```python
from build123d import *

# Parameters (mm, degrees)
SKETCH1_R           = 1.65
BOSS_EXTRUDE1_DEPTH = 2
SKETCH2_R           = 1.25
BOSS_EXTRUDE2_DEPTH = 2
SKETCH3_R           = 7.5
CUT_EXTRUDE1_DEPTH  = 2
BOSS_EXTRUDE3_START = 2.65408
SKETCH4_R           = 2.5
SKETCH4_R_2         = 1.25
BOSS_EXTRUDE3_DEPTH = 2.65408
SKETCH5_R           = 1.797788616
SKETCH5_R_2         = 1.10000034
SKETCH5_R_3         = 2.012466026
SKETCH5_R_4         = 1.729091626
SKETCH5_R_5         = 1.81324602
SKETCH5_R_6         = 1.075
BOSS_EXTRUDE4_DEPTH = 4.65408
CHAMFER1_SIZE       = 1.714507845
CHAMFER1_SIZE_2     = 0.15


with BuildPart() as part:
    # Sketch1 → Boss-Extrude1 (new body)
    with BuildSketch(Plane.XY):
        with BuildLine():
            Line((24.04163056, 18.384776311), (9.309167823, 3.652313574))
            ThreePointArc((9.309167823, 3.652313574), (9.985739131, -0.533867035), (8.866689125, -4.624048438))
            Line((8.866689125, -4.624048438), (23.334523779, -19.091883092))
            ThreePointArc((23.334523779, -19.091883092), (23.334523779, -23.334523779), (19.091883092, -23.334523779))
            Line((19.091883092, -23.334523779), (4.624048438, -8.866689125))
            ThreePointArc((4.624048438, -8.866689125), (0.533867035, -9.985739131), (-3.652313574, -9.309167823))
            Line((-3.652313574, -9.309167823), (-18.384776311, -24.04163056))
            ThreePointArc((-18.384776311, -24.04163056), (-24.04163056, -24.04163056), (-24.04163056, -18.384776311))
            Line((-24.04163056, -18.384776311), (-9.309167823, -3.652313574))
            ThreePointArc((-9.309167823, -3.652313574), (-9.985739131, 0.533867035), (-8.866689125, 4.624048438))
            Line((-8.866689125, 4.624048438), (-23.334523779, 19.091883092))
            ThreePointArc((-23.334523779, 19.091883092), (-23.334523779, 23.334523779), (-19.091883092, 23.334523779))
            Line((-19.091883092, 23.334523779), (-4.624048438, 8.866689125))
            ThreePointArc((-4.624048438, 8.866689125), (-0.533867035, 9.985739131), (3.652313574, 9.309167823))
            Line((3.652313574, 9.309167823), (18.384776311, 24.04163056))
            ThreePointArc((18.384776311, 24.04163056), (24.04163056, 24.04163056), (24.04163056, 18.384776311))
        make_face()
        with Locations((21.213203436, -21.213203436)):
            Circle(SKETCH1_R, mode=Mode.SUBTRACT)
        with Locations((21.213203436, 21.213203436)):
            Circle(SKETCH1_R, mode=Mode.SUBTRACT)
        with Locations((-21.213203436, 21.213203436)):
            Circle(SKETCH1_R, mode=Mode.SUBTRACT)
        with Locations((-21.213203436, -21.213203436)):
            Circle(SKETCH1_R, mode=Mode.SUBTRACT)
    extrude(amount=BOSS_EXTRUDE1_DEPTH)

    # Sketch2 → Boss-Extrude2 (add)
    with BuildSketch(Plane.XY.offset(2)):
        with BuildLine():
            Line((-2.135460216, 12.713781538), (12.713781227, -2.135459905))
            ThreePointArc((12.713781227, -2.135459905), (13.446014274, -3.903226858), (12.713781227, -5.670993811))
            Line((12.713781227, -5.670993811), (3.874947975, -14.509827063))
            ThreePointArc((3.874947975, -14.509827063), (2.107181022, -15.24206011), (0.339414069, -14.509827063))
            Line((0.339414069, -14.509827063), (-14.509827374, 0.33941438))
            ThreePointArc((-14.509827374, 0.33941438), (-15.242060421, 2.107181333), (-14.509827374, 3.874948286))
            Line((-14.509827374, 3.874948286), (-5.670994122, 12.713781538))
            ThreePointArc((-5.670994122, 12.713781538), (-3.903227169, 13.446014585), (-2.135460216, 12.713781538))
        make_face()
        with Locations((-3.903227169, 10.946014585)):
            Circle(SKETCH2_R, mode=Mode.SUBTRACT)
        with Locations((10.946014274, -3.903226858)):
            Circle(SKETCH2_R, mode=Mode.SUBTRACT)
        with Locations((2.107181022, -12.74206011)):
            Circle(SKETCH2_R, mode=Mode.SUBTRACT)
        with Locations((-12.742060421, 2.107181333)):
            Circle(SKETCH2_R, mode=Mode.SUBTRACT)
    extrude(amount=-BOSS_EXTRUDE2_DEPTH)

    # Sketch3 → Cut-Extrude1 (cut)
    with BuildSketch(Plane.XY.offset(2)):
        Circle(SKETCH3_R)
    extrude(amount=-CUT_EXTRUDE1_DEPTH, mode=Mode.SUBTRACT)

    # Sketch4 → Boss-Extrude3 (add)
    # profile 1 of 4: a face of its own
    with BuildSketch(Plane.XY.offset(2).offset(BOSS_EXTRUDE3_START)):
        with Locations(Location((-3.903227169, 10.946014585, 0), (0, 0, 45))):
            Circle(SKETCH4_R)
        with Locations((-3.903227169, 10.946014585)):
            Circle(SKETCH4_R_2, mode=Mode.SUBTRACT)
    # profile 2 of 4: a face of its own
    with BuildSketch(Plane.XY.offset(2).offset(BOSS_EXTRUDE3_START)):
        with Locations(Location((-12.742060421, 2.107181333, 0), (0, 0, 135))):
            Circle(SKETCH4_R)
        with Locations((-12.742060421, 2.107181333)):
            Circle(SKETCH4_R_2, mode=Mode.SUBTRACT)
    # profile 3 of 4: a face of its own
    with BuildSketch(Plane.XY.offset(2).offset(BOSS_EXTRUDE3_START)):
        with Locations(Location((10.946014274, -3.903226858, 0), (0, 0, 45))):
            Circle(SKETCH4_R)
        with Locations((10.946014274, -3.903226858)):
            Circle(SKETCH4_R_2, mode=Mode.SUBTRACT)
    # profile 4 of 4: a face of its own
    with BuildSketch(Plane.XY.offset(2).offset(BOSS_EXTRUDE3_START)):
        with Locations(Location((2.107181022, -12.74206011, 0), (0, 0, 315))):
            Circle(SKETCH4_R)
        with Locations((2.107181022, -12.74206011)):
            Circle(SKETCH4_R_2, mode=Mode.SUBTRACT)
    extrude(amount=-BOSS_EXTRUDE3_DEPTH)

    # Sketch5 → Boss-Extrude4 (add)
    # profile 1 of 4: a face of its own
    with BuildSketch(Plane.XY.offset(4.65408)):
        with Locations((10.946014274, -3.903226858)):
            Circle(SKETCH5_R)
        with Locations((10.946014274, -3.903226858)):
            Circle(SKETCH5_R_2, mode=Mode.SUBTRACT)
    # profile 2 of 4: a face of its own
    with BuildSketch(Plane.XY.offset(4.65408)):
        with Locations((2.107181022, -12.74206011)):
            Circle(SKETCH5_R_3)
        with Locations((2.107181022, -12.74206011)):
            Circle(SKETCH5_R_2, mode=Mode.SUBTRACT)
    # profile 3 of 4: a face of its own
    with BuildSketch(Plane.XY.offset(4.65408)):
        with Locations((-12.742060421, 2.107181333)):
            Circle(SKETCH5_R_4)
        with Locations((-12.742060421, 2.107181333)):
            Circle(SKETCH5_R_2, mode=Mode.SUBTRACT)
    # profile 4 of 4: a face of its own
    with BuildSketch(Plane.XY.offset(4.65408)):
        with Locations((-3.903227169, 10.946014585)):
            Circle(SKETCH5_R_5)
        with Locations((-3.903227169, 10.946014585)):
            Circle(SKETCH5_R_6, mode=Mode.SUBTRACT)
    extrude(amount=-BOSS_EXTRUDE4_DEPTH)

    # Chamfer1
    # the kernel refuses this chamfer: 1.714507845, 0.15 mm, written as the material it takes off along each edge
    with BuildSketch(Plane(origin=(10.946014274, -3.903226858, 4.65408), x_dir=(1, 0, 0), z_dir=(0, -1, 0))) as chamfer1_piece_1:
        Polygon((1.10000034, -CHAMFER1_SIZE), (1.10000034 + CHAMFER1_SIZE_2, 0), (1.10000034, 0), align=None)
    revolve(axis=Axis((10.946014274, -3.903226858, 4.65408), (0, 0, 1)), mode=Mode.SUBTRACT)
    with BuildSketch(Plane(origin=(2.107181022, -12.74206011, 4.65408), x_dir=(1, 0, 0), z_dir=(0, -1, 0))) as chamfer1_piece_2:
        Polygon((1.10000034, -CHAMFER1_SIZE), (1.10000034 + CHAMFER1_SIZE_2, 0), (1.10000034, 0), align=None)
    revolve(axis=Axis((2.107181022, -12.74206011, 4.65408), (0, 0, 1)), mode=Mode.SUBTRACT)
    with BuildSketch(Plane(origin=(-12.742060421, 2.107181333, 4.65408), x_dir=(1, 0, 0), z_dir=(0, -1, 0))) as chamfer1_piece_3:
        Polygon((1.10000034, -CHAMFER1_SIZE), (1.10000034 + CHAMFER1_SIZE_2, 0), (1.10000034, 0), align=None)
    revolve(axis=Axis((-12.742060421, 2.107181333, 4.65408), (0, 0, 1)), mode=Mode.SUBTRACT)
    with BuildSketch(Plane(origin=(-3.903227169, 10.946014585, 4.65408), x_dir=(1, 0, 0), z_dir=(0, -1, 0))) as chamfer1_piece_4:
        Polygon((1.075, -CHAMFER1_SIZE), (1.075 + CHAMFER1_SIZE_2, 0), (1.075, 0), align=None)
    revolve(axis=Axis((-3.903227169, 10.946014585, 4.65408), (0, 0, 1)), mode=Mode.SUBTRACT)


solid = part.part
```
Model file for the job. Use its own axes, mm. A direction names the side the tool comes from. Give positions to 0.01 mm unless a question says otherwise; leave off trailing zeros. Write each loop counter-clockwise with the first axis right and the second up, starting at its lowest first coordinate (ties: lowest second). Pieces come first, ordered by that corner, then holes. Notation, with made-up numbers: (-24.75, -38) -> (33.25, -38) arc R13 cw to (33.25, -21) -> close; hole circle Ø1 at (42, 32). An arc over 180 degrees is marked (long way). Use CSV: the item, a comma, the result in double quotes. Start each with the question number.
1) Tool access for faces 5 (the flat face through (-17.24, 13, 0.99)), 6 (the flat face through (-6.381, 12.004, 1.014)), 7 (the flat face through (-1.93, -12.24, 1.01)), 8 (the cylindrical face through (9.76, 2.17, 0.99)): list every direction of +Z, -Z, +X, -X, +Y, -Y with a clear straight run to the whole face (end or side of a thin tool).
2) Pin check, flat tip, straight feed: P1, Ø10, axis at x = 11, y = 10.5, coming from the +Z side. Stop position of the tip, or through.
3) Cut at C-C on y = -17.5. List the corners of the cut face in (x, z), plus the area to 3 significant figures.
4) Cut at A-A on z = 4. List the corners of the cut face in (x, y).
5) Cut at B-B on x = -22. List the corners of the cut face in (y, z), plus the area to 3 significant figures.
6) Cut at D-D on x = 17. List the corners of the cut face in (y, z), plus the area to 3 significant figures.
7) Drill centre lines: L1, parallel to Y at x = 3, z = 1.1; L2, parallel to Z at x = 18, y = -20; L3, parallel to X at y = 2, z = 2.9. Where is each one in solid material? Low to high.
8) Two-plate mould, pull along Y, no slides. Class faces 1 (the conical face through (9.788, -3.852, 3.618)), 2 (the flat face through (-13.17, 17.41, 0.99)), 3 (the cylindrical face through (-21.43, 22.85, 0.99)), 4 (the flat face through (5.495, -12.889, 1.014)): released by +Y, released by -Y, zero draft, split by the parting line, or undercut.
Final values:
1,face 5,"+Z, -Z, -X"
1,face 6,"+Z, -Z, +Y"
1,face 7,"+Z, -Z, -Y"
1,face 8,"+Z, -Z, +X"
2,P1,"stops at z = 2"
3,outline,"(-23.16, 0) -> (-11.84, 0) -> (-11.84, 2) -> (-23.16, 2) -> close; (13.26, 0) -> (21.74, 0) -> (21.74, 2) -> (13.26, 2) -> close"
3,area,"39.6 mm2"
4,outline,"circle Ø5 at (-12.74, 2.11); circle Ø5 at (-3.9, 10.95); circle Ø5 at (2.11, -12.74); circle Ø5 at (10.95, -3.9); hole circle Ø2.39 at (-12.74, 2.11); hole circle Ø2.34 at (-3.9, 10.95); hole circle Ø2.39 at (2.11, -12.74); hole circle Ø2.39 at (10.95, -3.9)"
5,outline,"(-25.14, 0) -> (-22.66, 0) -> (-22.66, 2) -> (-25.14, 2) -> close; (-19.76, 0) -> (-16.34, 0) -> (-16.34, 2) -> (-19.76, 2) -> close; (17.76, 0) -> (19.76, 0) -> (19.76, 2) -> (17.76, 2) -> close; (22.66, 0) -> (24.11, 0) -> (24.11, 2) -> (22.66, 2) -> close"
5,area,"18.7 mm2"
6,outline,"(-21.24, 0) -> (-12.76, 0) -> (-12.76, 2) -> (-21.24, 2) -> close; (11.34, 0) -> (22.66, 0) -> (22.66, 2) -> (11.34, 2) -> close"
6,area,"39.6 mm2"
7,L1,"y = -15.08 to -13.38, -12.1 to -6.87, 6.87 to 9.54"
7,L2,"z = 0 to 2"
7,L3,"x = -15.24 to -13.84, -11.65 to -10.24"
8,face 1,"undercut"
8,face 2,"released by +Y"
8,face 3,"undercut"
8,face 4,"released by -Y"
